Source: CAD feature listing. Evaluate the final solid. Frame: model axes, mm. Face numbers are marked on the shaded views. A direction names the side the tool comes from. Give positions to 0.01 mm unless a question says otherwise; leave off trailing zeros. Order: outer loops, then holes, each group sorted by start corner. A loop starts at its lowest first (then second) coordinate and runs counter-clockwise, first axis right, second up.
```python
from build123d import *

# Parameters (mm, degrees)
BOSS_EXTRU_1_DEPTH                             = 171
FRAISAGE_POUR_VIS_T_TE_FRAIS_E_M31_D           = 3.2
FRAISAGE_POUR_VIS_T_TE_FRAIS_E_M31_DEPTH       = 4
FRAISAGE_POUR_VIS_T_TE_FRAIS_E_M31_CSINK_D     = 6.3
FRAISAGE_POUR_VIS_T_TE_FRAIS_E_M31_CSINK_ANGLE = 90
D_GAGEMENT_M1_61_D                             = 1.7
D_GAGEMENT_M1_61_DEPTH                         = 4
ENL_V_MAT_EXTRU_1_DEPTH                        = 4
ENL_V_MAT_EXTRU_2_DEPTH                        = 31.75
ENL_V_MAT_EXTRU_2_DEPTH_BACK                   = 5


with BuildPart() as part:
    # Esquisse1 → Boss.-Extru.1 (new body)
    with BuildSketch(Plane.XY):
        with BuildLine():
            Line((0, 0), (-25, 0))
            ThreePointArc((-25, 0), (-32.071067812, 2.928932188), (-35, 10))
            Line((-35, 10), (-35, 45))
            Line((-35, 45), (-31, 45))
            Line((-31, 45), (-31, 10))
            ThreePointArc((-31, 10), (-29.242640687, 5.757359313), (-25, 4))
            Line((-25, 4), (0, 4))
            Line((0, 4), (0, 0))
        make_face()
    extrude(amount=BOSS_EXTRU_1_DEPTH)

    # Fraisage pour vis à tête fraisée M31
    with Locations(Plane(origin=(-31, 0, 0), x_dir=(0, 0, 1), z_dir=(1, 0, 0))):
        with Locations((4, -41), (167, -41)):
            CounterSinkHole(FRAISAGE_POUR_VIS_T_TE_FRAIS_E_M31_D / 2, FRAISAGE_POUR_VIS_T_TE_FRAIS_E_M31_CSINK_D / 2, depth=FRAISAGE_POUR_VIS_T_TE_FRAIS_E_M31_DEPTH, counter_sink_angle=FRAISAGE_POUR_VIS_T_TE_FRAIS_E_M31_CSINK_ANGLE)

    # Dégagement M1.61
    with Locations(Plane(origin=(0, 0, 0), x_dir=(-1, 0, 0), z_dir=(0, -1, 0))):
        with Locations((20.75, -65), (20.75, -106), (4.25, -106), (4.25, -65)):
            Hole(D_GAGEMENT_M1_61_D / 2, depth=D_GAGEMENT_M1_61_DEPTH)

    # Esquisse6 → Enlèv. mat.-Extru.1 (cut)
    with BuildSketch(Plane.XZ):
        with BuildLine():
            Line((-35, 61), (-3.25, 61))
            ThreePointArc((-3.25, 61), (-1.128679656, 61.878679656), (-0.25, 64))
            Line((-0.25, 64), (-0.25, 67))
            ThreePointArc((-0.25, 67), (-0.835786438, 68.414213562), (-2.25, 69))
            Line((-2.25, 69), (-3.750142858, 69))
            ThreePointArc((-3.750142858, 69), (-5.097923909, 68.680202649), (-6.15836042, 67.788990826))
            ThreePointArc((-6.15836042, 67.788990826), (-17.832822404, 66.671534919), (-17.754587156, 78.399094322))
            ThreePointArc((-17.754587156, 78.399094322), (-17.012643745, 79.411706018), (-16.75, 80.639256723))
            Line((-16.75, 80.639256723), (-16.75, 90.360743277))
            ThreePointArc((-16.75, 90.360743277), (-17.012643745, 91.588293982), (-17.754587156, 92.600905678))
            ThreePointArc((-17.754587156, 92.600905678), (-17.832822404, 104.328465081), (-6.15836042, 103.211009174))
            ThreePointArc((-6.15836042, 103.211009174), (-5.097923909, 102.319797351), (-3.750142858, 102))
            Line((-3.750142858, 102), (-2.25, 102))
            ThreePointArc((-2.25, 102), (-0.835786438, 102.585786438), (-0.25, 104))
            Line((-0.25, 104), (-0.25, 107))
            ThreePointArc((-0.25, 107), (-1.128679656, 109.121320344), (-3.25, 110))
            Line((-3.25, 110), (-35, 110))
            Line((-35, 110), (-35, 171))
            Line((-35, 171), (0, 171))
            Line((0, 171), (0, 0))
            Line((0, 0), (-35, 0))
            Line((-35, 0), (-35, 61))
        make_face()
        with BuildLine():
            Line((-18.75, 89.5), (-18.75, 81.5))
            ThreePointArc((-18.75, 81.5), (-20.75, 79.5), (-22.75, 81.5))
            Line((-22.75, 81.5), (-22.75, 89.5))
            ThreePointArc((-22.75, 89.5), (-20.75, 91.5), (-18.75, 89.5))
        make_face()
    extrude(amount=-ENL_V_MAT_EXTRU_1_DEPTH, mode=Mode.SUBTRACT)

    # Esquisse7 → Enlèv. mat.-Extru.2 (cut, two sides)
    with BuildSketch(Plane(origin=(-31, 0, 0), x_dir=(0, 0, -1), z_dir=(1, 0, 0))) as enl_v_mat_extru_2_sk:
        with BuildLine():
            ThreePointArc((-4, 45), (-1.171572875, 43.828427125), (0, 41))
            Line((0, 41), (0, 45))
            Line((0, 45), (-4, 45))
        make_face()
        with BuildLine():
            Line((0, 4), (0, 41))
            ThreePointArc((0, 41), (-1.171572875, 38.171572875), (-4, 37))
            Line((-4, 37), (-31, 37))
            ThreePointArc((-31, 37), (-52.213203436, 28.213203436), (-61, 7))
            Line((-61, 7), (-61, 4))
            Line((-61, 4), (0, 4))
        make_face()
        with BuildLine():
            ThreePointArc((-167, 37), (-169.828427125, 38.171572875), (-171, 41))
            Line((-171, 41), (-171, 4))
            Line((-171, 4), (-110, 4))
            Line((-110, 4), (-110, 7))
            ThreePointArc((-110, 7), (-118.786796564, 28.213203436), (-140, 37))
            Line((-140, 37), (-167, 37))
        make_face()
        with BuildLine():
            Line((-171, 45), (-171, 41))
            ThreePointArc((-171, 41), (-169.828427125, 43.828427125), (-167, 45))
            Line((-167, 45), (-171, 45))
        make_face()
        with BuildLine():
            Line((-65.985711369, 37), (-105.014288631, 37))
            ThreePointArc((-105.014288631, 37), (-109.460347769, 34.287478555), (-109.082394604, 29.093023256))
            ThreePointArc((-109.082394604, 29.093023256), (-104.093528666, 19.438863146), (-102.041125553, 8.76744186))
            ThreePointArc((-102.041125553, 8.76744186), (-100.498870029, 5.383178834), (-97.04653681, 4))
            Line((-97.04653681, 4), (-73.95346319, 4))
            ThreePointArc((-73.95346319, 4), (-70.501129971, 5.383178834), (-68.958874447, 8.76744186))
            ThreePointArc((-68.958874447, 8.76744186), (-66.906471334, 19.438863146), (-61.917605396, 29.093023256))
            ThreePointArc((-61.917605396, 29.093023256), (-61.539652231, 34.287478555), (-65.985711369, 37))
        make_face()
    extrude(amount=ENL_V_MAT_EXTRU_2_DEPTH, mode=Mode.SUBTRACT)
    extrude(enl_v_mat_extru_2_sk.sketch, amount=-ENL_V_MAT_EXTRU_2_DEPTH_BACK, mode=Mode.SUBTRACT)


solid = part.part
```
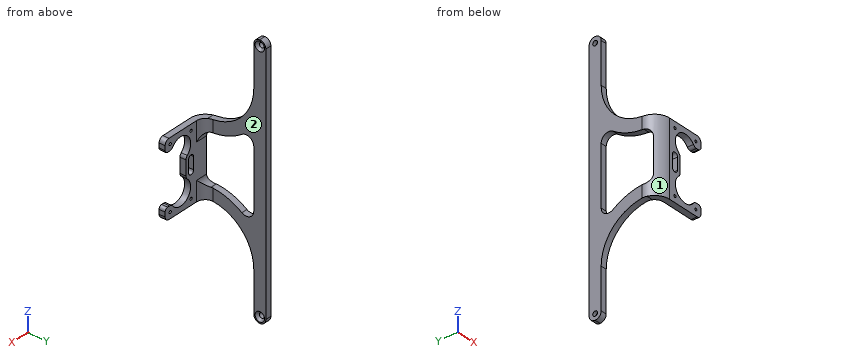
1) Section query D-D, the plane z = 125.5. Return the cut outline in (x, y), and give its area (3 significant figures).
Report:
outline: (-35, 33.26) - (-31, 33.26) - (-31, 45) - (-35, 45) - close
area: 46.9 mm2
2) Section query C-C, the plane x = -9. Return the cut outline in (y, z), and give its area (3 significant figures).
Report:
outline: (0, 61) - (4, 61) - (4, 65.42) - (0, 65.42) - close; (0, 105.58) - (4, 105.58) - (4, 110) - (0, 110) - close
area: 35.3 mm2
3) Material intervals for L1, parallel to Z at x = -20.75, y = 1.5; L2, parallel to Z at x = -4.25, y = 2.85; L3, parallel to Z at x = -12.5, y = 1.65, sorted ascending.
Report:
L1: z = 61 to 64.15, 65.85 to 79.5, 91.5 to 105.15, 106.85 to 110
L2: z = 61 to 64.15, 65.85 to 68.96, 102.04 to 105.15, 106.85 to 110
L3: z = 61 to 64.6, 106.4 to 110
4) Reachability of the marked faces 1 and 2 from +Z, -Z, +X, -X, +Y, -Y: full face, straight path, thin tool, end or side. Return the list, or none.
Report:
face 1: +Z, -Z, -X, -Y
face 2: +Z, -Z, +X, +Y
5) Section query B-B, the plane y = 21. Return the cut outline in (x, z).
Report:
outline: (-35, 57.53) - (-31, 57.53) - (-31, 66.33) - (-35, 66.33) - close; (-35, 104.67) - (-31, 104.67) - (-31, 113.47) - (-35, 113.47) - close
6) Section query A-A, the plane z = 98.5. Return the cut outline in (x, y).
Report:
outline: (-35, 37) - (-31, 37) - (-31, 45) - (-35, 45) - close; (-33.16, 4.22) arc R10 ccw to (-25, 0) - (-20.4, 0) - (-20.4, 4) - (-25, 4) arc R6 cw to (-26.6, 4.22) - close
7) Pin query (flat end, axial travel): pin 1 (1.2 mm diameter, centred on x = -3, y = 2.5, fed in from -Z); pin 2 (1.7 mm diameter, centred on x = -2.5, y = 1.5, fed in from +Z); pin 3 (1.2 mm diameter, centred on x = -33.5, z = 81.5, fed in from -Y). Return the tip coordinate at first contact, or that it passes through.
Report:
pin 1: stops at z = 61
pin 2: stops at z = 110
pin 3: stops at y = 3.87
